from build123d import *

# Parameters (mm, degrees)
SKETCH2_W               = 34
SKETCH2_H               = 1
EXTRUDE1_DEPTH          = 22
EXTRUDE1_2_DEPTH        = 22
EXTRUDE1_3_DEPTH        = 22
EXTRUDE1_4_DEPTH        = 22
CUT_EXTRUDE1_DEPTH      = 29.670542374
CUT_EXTRUDE1_DEPTH_BACK = 29.670542374
EXTRUDE2_DEPTH          = 1
EXTRUDE3_REACH          = 31.598


with BuildPart() as part:
    # Sketch2 → Extrude1 (new body)
    with BuildSketch(Plane.XY):
        with Locations((0, 13.75)):
            Rectangle(SKETCH2_W, SKETCH2_H)
    extrude(amount=EXTRUDE1_DEPTH)


with BuildPart() as body_2:
    # Sketch2 → Extrude1 2 (new body)
    with BuildSketch(Plane.XY):
        with Locations((0, 11.75)):
            Rectangle(SKETCH2_W, SKETCH2_H)
    extrude(amount=EXTRUDE1_2_DEPTH)


with BuildPart() as body_3:
    # Sketch2 → Extrude1 3 (new body)
    with BuildSketch(Plane.XY):
        with Locations((0, 9.75)):
            Rectangle(SKETCH2_W, SKETCH2_H)
    extrude(amount=EXTRUDE1_3_DEPTH)


with BuildPart() as body_4:
    # Sketch2 → Extrude1 4 (new body)
    with BuildSketch(Plane.XY):
        with Locations((0, 7.75)):
            Rectangle(SKETCH2_W, SKETCH2_H)
    extrude(amount=EXTRUDE1_4_DEPTH)


with BuildPart() as cut_extrude1_tool:
    # Sketch3 → Cut-Extrude1 (new, two sides: drawn at the far end of the back side and taken through both)
    with BuildSketch(Plane(origin=(0, 14.25, 0), x_dir=(1, 0, 0), z_dir=(0, 1, 0)).offset(-CUT_EXTRUDE1_DEPTH_BACK)):
        with BuildLine():
            Line((-102.195874551, -1.64205818), (-17, -5.829814285))
            ThreePointArc((-17, -5.829814285), (-1.114330758, -10.529941826), (10.839055861, -22))
            Line((10.839055861, -22), (56.687802572, -93.928900776))
            Line((56.687802572, -93.928900776), (-28.997329883, -241.446884233))
            Line((-28.997329883, -241.446884233), (-187.881007007, -149.160041637))
            Line((-187.881007007, -149.160041637), (-102.195874551, -1.64205818))
        make_face()
    extrude(amount=CUT_EXTRUDE1_DEPTH + CUT_EXTRUDE1_DEPTH_BACK)


with BuildPart() as part_1:
    add(part.part)

    # Cut-Extrude1: cut by cut_extrude1_tool
    add(cut_extrude1_tool.part, mode=Mode.SUBTRACT)



with BuildPart() as body_2_1:
    add(body_2.part)

    # Cut-Extrude1: cut by cut_extrude1_tool
    add(cut_extrude1_tool.part, mode=Mode.SUBTRACT)


with BuildPart() as body_3_1:
    add(body_3.part)

    # Cut-Extrude1: cut by cut_extrude1_tool
    add(cut_extrude1_tool.part, mode=Mode.SUBTRACT)


with BuildPart() as body_4_1:
    add(body_4.part)

    # Cut-Extrude1: cut by cut_extrude1_tool
    add(cut_extrude1_tool.part, mode=Mode.SUBTRACT)


with BuildPart() as part_2:
    add(part_1.part)

    add(body_2_1.part)  # Extrude2 merges body 2

    add(body_3_1.part)  # Extrude2 merges body 3

    add(body_4_1.part)  # Extrude2 merges body 4
    # Sketch1 → Extrude2 (add)
    with BuildSketch(Plane.XY):
        Polygon((-16, 6), (-18, 6), (-18, 15.5), (18, 15.5), (18, 6), (16, 6), align=None)
    extrude(amount=EXTRUDE2_DEPTH)

    # Extrude3: up to this face of the body (flat: up to its plane)
    extrude3_end = Plane(part_2.part.faces().sort_by_distance((4.784093831, 7.25, 8.43063068))[0])
    # Sketch4 → Extrude3 (add, up to the picked face)
    with BuildSketch(Plane(origin=(0, 14.25, 0), x_dir=(1, 0, 0), z_dir=(0, 1, 0)), mode=Mode.PRIVATE) as extrude3_sk1:
        with BuildLine():
            Line((17, -13.384444495), (17, -1))
            Line((17, -1), (2.315156907, -1))
            ThreePointArc((2.315156907, -1), (10.32529612, -6.40047667), (17, -13.384444495))
        make_face()
    extrude3_tool1 = split(extrude(extrude3_sk1.sketch, amount=-EXTRUDE3_REACH, mode=Mode.PRIVATE), bisect_by=extrude3_end, keep=Keep.BOTH, mode=Mode.PRIVATE)
    add(extrude3_tool1.solids().sort_by(Axis((12.478382, 14.25, 4.828977), (0, -1, 0)))[0])


solid = part_2.part
For this review, take the finished solid that the model builds, in its own axes (mm). A direction names the side the tool comes from. Give positions to 0.01 mm unless a question says otherwise; leave off trailing zeros. Loops run counter-clockwise (first coordinate to the right, second up) from the corner with the lowest first, then second, coordinate; pieces in that order, holes last. Notation, with made-up numbers: (25.25, 49) - (82.25, 49) arc R9 ccw to (82.25, 60) - close; hole circle Ø2 at (-16.5, -32). An arc over 180 degrees is marked (long way). Write each question's results on one line, items separated by ' | '.
(1) For pin 1 Ø5 at (y, z) = (14, 4.5) entering from -X; pin 2 Ø10.5 at (x, z) = (-5.5, 11) entering from -Y; pin 3 Ø6.5 at (x, z) = (4, 12) entering from +Y, all flat-tipped, find the tip position at first contact; note any pin that passes through.
Conclusion:
pin 1: x = -17 | pin 2: y = 7.25 | pin 3: y = 14.25
(2) Take a section at B-B (y = 9.75). Give the boundary of the cut face in (x, z).
Conclusion:
outline: (-18, 0) - (18, 0) - (18, 1) - (17, 1) - (17, 22) - (10.84, 22) arc R35.05 cw to (-17, 5.83) - (-17, 1) - (-18, 1) - close
(3) Take a section at C-C (x = -0.5). Give the boundary of the cut face in (y, z).
Conclusion:
outline: (6, 0) - (15.5, 0) - (15.5, 1) - (14.25, 1) - (14.25, 10.9) - (13.25, 10.9) - (13.25, 1) - (12.25, 1) - (12.25, 10.9) - (11.25, 10.9) - (11.25, 1) - (10.25, 1) - (10.25, 10.9) - (9.25, 10.9) - (9.25, 1) - (8.25, 1) - (8.25, 10.9) - (7.25, 10.9) - (7.25, 1) - (6, 1) - close
(4) Take a section at A-A (z = 15.25). Give the boundary of the cut face in (x, y).
Conclusion:
outline: (5.23, 7.25) - (17, 7.25) - (17, 8.25) - (5.23, 8.25) - close; (5.23, 9.25) - (17, 9.25) - (17, 10.25) - (5.23, 10.25) - close; (5.23, 11.25) - (17, 11.25) - (17, 12.25) - (5.23, 12.25) - close; (5.23, 13.25) - (17, 13.25) - (17, 14.25) - (5.23, 14.25) - close
(5) For faces 1 (the flat face through (17, 11, 9)), 2 (the flat face through (4, 12.25, 9)), 3 (the flat face through (4, 7.25, 9)), list the 3-axis set-ups (+Z, -Z, +X, -X, +Y, -Y) from which the entire face can be reached by the end or side of a thin tool; tool diameter is ignored.
Conclusion:
face 1: +Z, +X, +Y, -Y | face 2: +Z, -X | face 3: +Z, +X, -X, -Y
(6) For line 1 along Y through (x, z) = (2, 5.5); line 2 along X through (y, z) = (13.5, 1.75); line 3 along Z through (x, y) = (-14, 8.5), list the stretches that pass through material, from the lowest coordinate up.
Conclusion:
line 1: 7.25 to 8.25, 9.25 to 10.25, 11.25 to 12.25, 13.25 to 14.25 | line 2: -17 to 17 | line 3: 0 to 1
(7) Take a section at D-D (z = 2.75). Give the boundary of the cut face in (x, y), then the cut area to 3 significant figures.
Conclusion:
outline: (-17, 7.25) - (17, 7.25) - (17, 14.25) - (-17, 14.25) - (-17, 13.25) - (5.34, 13.25) - (5.34, 12.25) - (-17, 12.25) - (-17, 11.25) - (5.34, 11.25) - (5.34, 10.25) - (-17, 10.25) - (-17, 9.25) - (5.34, 9.25) - (5.34, 8.25) - (-17, 8.25) - close | area: 171 mm^2
